The model under review builds one solid part; all positions refer to its coordinate system, in mm. A direction names the side the tool comes from. Round coordinates to 2 decimals unless told otherwise and drop trailing zeros. Loops run counter-clockwise (first coordinate to the right, second up) from the corner with the lowest first, then second, coordinate; pieces in that order, holes last. Notation, with made-up numbers: (2, 10.25) -> (12, 10.25) arc R30 ccw to (12, 37.25) -> close; hole circle Ø8 at (-12, -6). An arc over 180 degrees is marked (long way). Use a Markdown table: item, result. Add a question column.
1) Consider section A-A on x = 0. State how many separate pieces and enclosed holes the cut face has, plus the area to 3 significant figures.
2) Wall thickness on probe 1 along Y at (x, z) = (0, -2.5); probe 2 along Y at (x, z) = (0, -10.25); probe 3 along Z at (x, y) = (7, 22.5): over which ranges is each line inside the solid? List them lowest first.
3) Mouldability with a two-part tool opening along Y and no side actions: class faces 4 (the cylindrical face through (-0.5, -11.3, -2)), 5 (the flat face through (-5, 9, 0)), 6 (the cylindrical face through (-4.336, -19.524, -9.86)), 7 (the cylindrical face through (-2.17, -9.76, -1.97)) as released by +Y, released by -Y, zero draft, split by the parting line, or undercut.
4) Consider section B-B on z = -6.25. Give the boundary of the cut face in (x, y).
5) For faces 1 (the cylindrical face through (-13.887, -10.648, -11.888)), 2 (the flat face through (5.9, -19.4, -20)), 3 (the cylindrical face through (11.252, -0.11, -2.028)), list the 3-axis set-ups (+Z, -Z, +X, -X, +Y, -Y) from which the entire face can be reached by the end or side of a thin tool; tool diameter is ignored.
6) Insertion check: pin 1 (6.5 mm diameter, centred on x = 0, y = -13.75, fed in from -Z); pin 2 (6 mm diameter, centred on x = -7.5, z = -9, fed in from +Y); pin 3 (4.5 mm diameter, centred on x = 0, y = 13.75, fed in from -Z); pin 4 (6 mm diameter, centred on x = 15.5, z = -15, fed in from +Y). Each pin has a flat end and moves straight along its axis. Give the tip position at first contact, or say it passes through.
7) Consider section C-C on z = -21. Give the boundary of the cut face in (x, y), plus the area to 3 significant figures.
from build123d import *

# Parameters (mm, degrees)
F0_R     = 20
F0_R_2   = 17.5
F1_DEPTH = 23
F0_R_3   = 10
F2_DEPTH = 4
F3_R     = 28.5
F3_R_2   = 20
F4_DEPTH = 3
F5_R     = 2.5
F6_DEPTH = 4.001
F7_SIZE  = 2.99999
F8_SIZE  = 3


# Not quite as in the source:
# - a fillet or chamfer is up to 0.001 mm smaller than in the source, because OpenCascade refuses the exact size


with BuildPart() as f1:
    # F0 (on Top) → F1 (new body)
    with BuildSketch(Plane.XY):
        Circle(F0_R)
        Circle(F0_R_2, mode=Mode.SUBTRACT)
    extrude(amount=-F1_DEPTH)

    # F0 (on Top) → F2 (join)
    with BuildSketch(Plane.XY):
        Circle(F0_R_2)
        Circle(F0_R_3, mode=Mode.SUBTRACT)
    extrude(amount=-F2_DEPTH)

    # F3 (on face) → F4 (join)
    with BuildSketch(Plane(origin=(0, 0, -23), x_dir=(1, 0, 0), z_dir=(0, 0, -1))):
        Circle(F3_R)
        Circle(F3_R_2, mode=Mode.SUBTRACT)
    extrude(amount=-F4_DEPTH)

    # F5 (on face) → F6 (cut, through all)
    with BuildSketch(Plane(origin=(0, 0, -4), x_dir=(1, 0, 0), z_dir=(0, 0, -1))):
        with Locations((0, 13.75)):
            Circle(F5_R)
        with Locations((-13.75, 0)):
            Circle(F5_R)
        with Locations((0, -13.75)):
            Circle(F5_R)
        with Locations((13.75, 0)):
            Circle(F5_R)
    extrude(amount=-F6_DEPTH, mode=Mode.SUBTRACT)

    # F7 (size 3 in the source; OpenCascade refuses exactly that, so slightly less here)
    f7_edges = [f1.edges().sort_by_distance(p)[0] for p in [
        (-28.5, 0, -23),
    ]]
    chamfer(f7_edges, length=F7_SIZE)

    # F8
    f8_edges = [f1.edges().sort_by_distance(p)[0] for p in [
        (-17.5, 0, -23),
    ]]
    chamfer(f8_edges, length=F8_SIZE)


solid = f1.part
Result set:
| question | item | result |
|---|---|---|
| 1 | separate pieces | 4 |
| 1 | enclosed holes | 0 |
| 1 | area | 168 mm2 |
| 2 | probe 1 | -20 to -16.25, -11.25 to -10, 10 to 11.25, 16.25 to 20 |
| 2 | probe 2 | -20 to -17.5, 17.5 to 20 |
| 2 | probe 3 | -23 to -20 |
| 3 | face 4 | undercut |
| 3 | face 5 | zero draft |
| 3 | face 6 | split by the parting line |
| 3 | face 7 | undercut |
| 4 | outline | circle Ø40 at (0, 0); hole circle Ø35 at (0, 0) |
| 5 | face 1 | -Z |
| 5 | face 2 | +Z |
| 5 | face 3 | +Z, -Z |
| 6 | pin 1 | z = -4 |
| 6 | pin 2 | y = 19.49 |
| 6 | pin 3 | through |
| 6 | pin 4 | y = 15.61 |
| 7 | outline | circle Ø55 at (0, 0); hole circle Ø37 at (0, 0) |
| 7 | area | 1,300 mm2 |
